from build123d import *

# Parameters (mm, degrees)
SKETCH1_W           = 40
SKETCH1_H           = 50
BOSS_EXTRUDE1_DEPTH = 10
SKETCH3_R           = 7
CUT_EXTRUDE1_DEPTH  = 55.772255751


with BuildPart() as part:
    # Sketch1 → Boss-Extrude1 (new, symmetric)
    with BuildSketch(Plane(origin=(0, 0, 0), x_dir=(0, 0, -1), z_dir=(1, 0, 0))):
        Rectangle(SKETCH1_W, SKETCH1_H)
        with BuildLine():
            Line((-5, 20), (5, 20))
            ThreePointArc((5, 20), (12.071067812, 17.071067812), (15, 10))
            Line((15, 10), (15, -10))
            ThreePointArc((15, -10), (12.071067812, -17.071067812), (5, -20))
            Line((5, -20), (-5, -20))
            ThreePointArc((-5, -20), (-12.071067812, -17.071067812), (-15, -10))
            Line((-15, -10), (-15, 10))
            ThreePointArc((-15, 10), (-12.071067812, 17.071067812), (-5, 20))
        make_face(mode=Mode.SUBTRACT)
    extrude(amount=BOSS_EXTRUDE1_DEPTH, both=True)

    # Sketch3 → Cut-Extrude1 (cut, through all)
    with BuildSketch(Plane(origin=(0, 25, 0), x_dir=(1, 0, 0), z_dir=(0, 1, 0))):
        with Locations(Location((0, 0, 0), (0, 0, 270))):
            Circle(SKETCH3_R)
    extrude(amount=-CUT_EXTRUDE1_DEPTH, mode=Mode.SUBTRACT)


solid = part.part
Verification items for the finished model (mm, model axes). A direction names the side the tool comes from. Round coordinates to 2 decimals unless told otherwise and drop trailing zeros. Write each loop counter-clockwise with the first axis right and the second up, starting at its lowest first coordinate (ties: lowest second). Pieces come first, ordered by that corner, then holes.
(1) Material ranges on line 1 (Z direction, x = -6.75, y = 6); line 2 (Y direction, x = -8.25, z = 0); line 3 (X direction, y = -21.95, z = 0), recorded low to high.
Returned:
line 1: z = -20 to -15, 15 to 20
line 2: y = -25 to -20, 20 to 25
line 3: x = -10 to -7, 7 to 10
(2) Mould release check, pull along Y, two halves, no side actions. Record for faces 3 (the flat face through (7, -25, 5)), 4 (the flat face through (0, 0, -20)), 5 (the flat face through (-8, 20, 0)), 6 (the flat face through (-8, -20, 0)): pulls with the +Y half, pulls with the -Y half, needs draft (parallel to the pull), parting line crosses it, or undercut.
Returned:
face 3: pulls with the -Y half
face 4: needs draft
face 5: undercut
face 6: undercut
(3) Section check B-B (x = 0). Enter the section's corners in (y, z).
Returned:
outline: (-25, -20) - (25, -20) - (25, -7) - (19.8, -7) arc R10 cw to (10, -15) - (-10, -15) arc R10 cw to (-19.8, -7) - (-25, -7) - close; (-25, 7) - (-19.8, 7) arc R10 cw to (-10, 15) - (10, 15) arc R10 cw to (19.8, 7) - (25, 7) - (25, 20) - (-25, 20) - close
(4) Access from +Z, -Z, +X, -X, +Y, -Y to the whole of each face (thin tool, end or side, straight path). Record for faces 1 (the cylindrical face through (0.14, -16.99, -12.15)), 2 (the flat face through (10, 0, 18)).
Returned:
face 1: +X, -X
face 2: +Z, -Z, +X, +Y, -Y
(5) Section check D-D (z = 0). Enter the section's corners in (x, y), plus the area to 3 significant figures.
Returned:
outline: (-10, -25) - (-7, -25) - (-7, -20) - (-10, -20) - close; (-10, 20) - (-7, 20) - (-7, 25) - (-10, 25) - close; (7, -25) - (10, -25) - (10, -20) - (7, -20) - close; (7, 20) - (10, 20) - (10, 25) - (7, 25) - close
area: 60.0 mm2
(6) Section check C-C (z = 13). Enter the section's corners in (x, y).
Returned:
outline: (-10, -25) - (10, -25) - (10, -16) - (-10, -16) - close; (-10, 16) - (10, 16) - (10, 25) - (-10, 25) - close
(7) Depth check by flat-ended pin: pin 1 Ø11 at (x, z) = (0, 0) entering from -Y. Enter the tip coordinate at first touch or a pass-through.
Returned:
pin 1: passes through
(8) Section check A-A (y = 2). Enter the section's corners in (x, z).
Returned:
outline: (-10, -20) - (10, -20) - (10, -15) - (-10, -15) - close; (-10, 15) - (10, 15) - (10, 20) - (-10, 20) - close
